Model file for the job. Use its own axes, mm. Coordinates: 2 decimals unless noted, no trailing zeros. Order: outer loops, then holes, each group sorted by start corner. A loop starts at its lowest first (then second) coordinate and runs counter-clockwise, first axis right, second up.
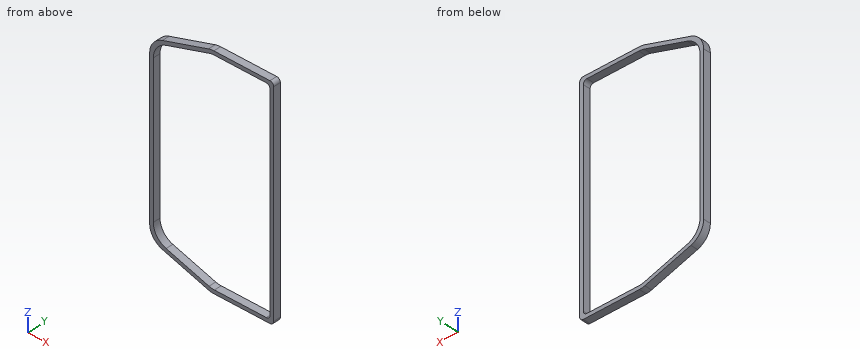
from build123d import *

# Parameters (mm, degrees)
EXTRUDE_1_DEPTH = 2
FILLET_1_R      = 5
FILLET_2_R      = 1
MIRROR_1_DEPTH  = 2


# Read off the part's stored shape, not the designer's step: the mirror step
with BuildPart() as part:
    # Sketch 1 → Extrude 1 (new body)
    with BuildSketch(Plane(origin=(0, 0, 0), x_dir=(1, 0, 0), z_dir=(0, 1, 0))):
        Polygon((0, 0), (0, 29), (-16, 29), (-32, 24), (-32, 0), (-33, 0), (-33, 24.735190913), (-16.152610923, 30), (1, 30), (1, 0), align=None)
    extrude(amount=EXTRUDE_1_DEPTH)

    # Fillet 1
    fillet_1_edges = [part.edges().sort_by_distance(p)[0] for p in [
        (-16, 1, -29),
        (-32, 1, -24),
        (-33, 1, -24.735190913),
        (-16.152610923, 1, -30),
    ]]
    fillet(fillet_1_edges, radius=FILLET_1_R)

    # Fillet 2
    fillet_2_edges = [part.edges().sort_by_distance(p)[0] for p in [
        (0, 1, -29),
        (1, 1, -30),
    ]]
    fillet(fillet_2_edges, radius=FILLET_2_R)

    # Mirror 1 outline → Mirror 1 (add)
    with BuildSketch(Plane(origin=(0, 0, 0), x_dir=(1, 0, 0), z_dir=(0, 1, 0))):
        with BuildLine():
            Line((1, -29), (1, 0))
            Line((1, 0), (0, 0))
            Line((0, 0), (0, -28))
            ThreePointArc((0, -28), (-0.292893219, -28.707106781), (-1, -29))
            Line((-1, -29), (-15.236945386, -29))
            ThreePointArc((-15.236945386, -29), (-15.991266454, -28.942772474), (-16.728320351, -28.77239989))
            Line((-16.728320351, -28.77239989), (-28.491374966, -25.096445323))
            ThreePointArc((-28.491374966, -25.096445323), (-31.028453477, -23.285727824), (-32, -20.324045433))
            Line((-32, -20.324045433), (-32, 0))
            Line((-32, 0), (-33, 0))
            Line((-33, 0), (-33, -21.059236346))
            ThreePointArc((-33, -21.059236346), (-32.028453477, -24.020918738), (-29.491374966, -25.831636237))
            Line((-29.491374966, -25.831636237), (-16.880931274, -29.77239989))
            ThreePointArc((-16.880931274, -29.77239989), (-16.143877377, -29.942772474), (-15.389556309, -30))
            Line((-15.389556309, -30), (0, -30))
            ThreePointArc((0, -30), (0.707106781, -29.707106781), (1, -29))
        make_face()
    extrude(amount=MIRROR_1_DEPTH)


solid = part.part
Q1. Cut at B-B, the plane y = 1.1. List the corners of the cut face in (x, z), plus the area to 3 significant figures.
Established:
outline: (-33, -21.06) arc R5 ccw to (-29.49, -25.83) - (-16.88, -29.77) arc R5 ccw to (-15.39, -30) - (0, -30) arc R1 ccw to (1, -29) - (1, 29) arc R1 ccw to (0, 30) - (-15.39, 30) arc R5 ccw to (-16.88, 29.77) - (-29.49, 25.83) arc R5 ccw to (-33, 21.06) - close; hole (-32, -20.32) arc R5 ccw to (-28.49, -25.1) - (-16.73, -28.77) arc R5 ccw to (-15.24, -29) - (-1, -29) arc R1 ccw to (0, -28) - (0, 28) arc R1 ccw to (-1, 29) - (-15.24, 29) arc R5 ccw to (-16.73, 28.77) - (-28.49, 25.1) arc R5 ccw to (-32, 20.32) - close
area: 175 mm2
Q2. Cut at C-C, the plane x = -14. List the corners of the cut face in (y, z), plus the area to 3 significant figures.
Established:
outline: (0, -30) - (2, -30) - (2, -29) - (0, -29) - close; (0, 29) - (2, 29) - (2, 30) - (0, 30) - close
area: 4.00 mm2
Q3. Probe line 1 (Z direction, x = -11.5, y = 1.3); line 2 (X direction, y = 0.2, z = -7); line 3 (Z direction, x = -28.5, y = 0.25). List the from-to ranges inside material, lowest first.
Established:
line 1: z = -30 to -29, 29 to 30
line 2: x = -33 to -32, 0 to 1
line 3: z = -26.14 to -25.09, 25.09 to 26.14
Q4. Cut at A-A, the plane z = 4.5. List the corners of the cut face in (x, y), plus the area to 3 significant figures.
Established:
outline: (-33, 0) - (-32, 0) - (-32, 2) - (-33, 2) - close; (0, 0) - (1, 0) - (1, 2) - (0, 2) - close
area: 4.00 mm2
